```python
from build123d import *

# Parameters (mm, degrees)
F0_W      = 177.038
F0_H      = 34.544
F1_DEPTH  = 6.35
F2_R      = 6.35
F3_DEPTH  = 6.351
F4_DEPTH  = 25.4
F6_W      = 130.2497221681
F6_H      = 6.35
F6_W_2    = 46.7882778319
F7_DEPTH  = 7.874
F9_DEPTH  = 25.4
F11_DEPTH = 25.4


with BuildPart() as f1:
    # F0 (on Front) → F1 (new body)
    with BuildSketch(Plane.XZ):
        with Locations((88.519, 17.272)):
            Rectangle(F0_W, F0_H)
    extrude(amount=F1_DEPTH)

    # F2 (on face) → F3 (cut, through all)
    with BuildSketch(Plane.XZ.offset(6.35)):
        with Locations((28.448, 14.732)):
            Circle(F2_R)
    extrude(amount=-F3_DEPTH, mode=Mode.SUBTRACT)

    # F2 (on face) → F4 (cut)
    with BuildSketch(Plane.XZ.offset(6.35)):
        with Locations((28.448, 14.732)):
            Circle(F2_R)
        with Locations((76.2, 11.684)):
            Circle(F2_R)
        with Locations((136.144, 2.3622)):
            Circle(F2_R)
    extrude(amount=-F4_DEPTH, mode=Mode.SUBTRACT)

    # F6 (on face) → F7 (join)
    with BuildSketch(Plane(origin=(0, 0, 0), x_dir=(1, 0, 0), z_dir=(0, 0, -1))):
        with Locations((65.124861084, 3.175)):
            Rectangle(F6_W, F6_H)
        with Locations((153.643861084, 3.175)):
            Rectangle(F6_W_2, F6_H)
    extrude(amount=F7_DEPTH)

    # F8 (on face) → F9 (cut)
    with BuildSketch(Plane.XZ.offset(6.35)):
        with BuildLine():
            Line((142.0382778319, 0), (130.2497221681, 0))
            ThreePointArc((130.2497221681, 0), (136.144, -3.9878), (142.0382778319, 0))
        make_face()
    extrude(amount=-F9_DEPTH, mode=Mode.SUBTRACT)

    # F10 (on face) → F11 (cut)
    with BuildSketch(Plane.XZ.offset(6.35)):
        Polygon((167.894, 34.544), (9.144, 34.544), (9.144, 23.8669347018), (86.614, 23.8669347018), (86.614, 13.97), (167.894, 13.97), align=None)
        Polygon((61.8659904612, 4.6831931899), (0, 3.9632934857), (0, -7.874), (62.0121114495, -7.874), align=None)
    extrude(amount=-F11_DEPTH, mode=Mode.SUBTRACT)


solid = f1.part
```
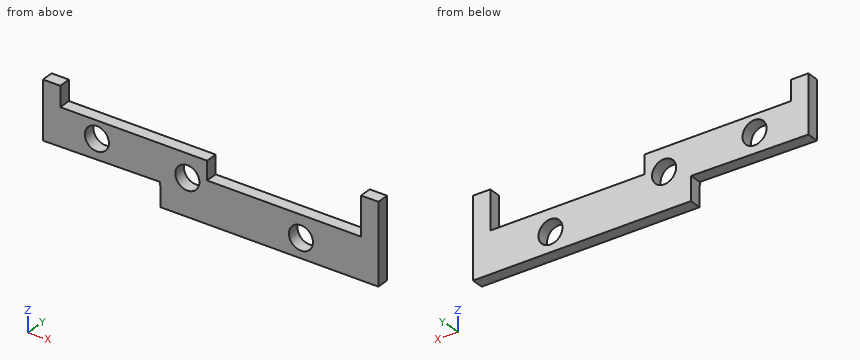
Geometry check sheet. Reference: the model listing, model coordinates, mm. Round coordinates to 2 decimals unless told otherwise and drop trailing zeros. Order: outer loops, then holes, each group sorted by start corner. A loop starts at its lowest first (then second) coordinate and runs counter-clockwise, first axis right, second up. Notation, with made-up numbers: (-14.75, -40) -> (0.25, -40) arc R24 cw to (0.25, -28) -> close; hole circle Ø7 at (42.25, 1.25). An arc over 180 degrees is marked (long way). Return JSON: item names as keys, results as strings. Group by question number.
Q1. Section check D-D, the plane x = 12.5. Record the boundary of the cut face in (y, z).
Q2. Section check C-C, the plane y = -3. Record the boundary of the cut face in (x, z).
Q3. Section check A-A, the plane z = 27.5. Record the boundary of the cut face in (x, y), plus the area to 3 significant figures.
Q4. Gauge pin test, flat ends, axial feed: pin 1 (3 mm diameter, centred on x = 81, y = -2, fed in from +Z); pin 2 (1.9 mm diameter, centred on x = 126, y = -4, fed in from +Z). Record the tip position at first contact, or that the pin passes through.
Q5. Material ranges on probe 1 along X at (y, z) = (-3.25, 27); probe 2 along X at (y, z) = (-3.5, 12); probe 3 along Z at (x, y) = (76.2, -2.25), recorded low to high. Write a range as from..to.
Q6. Section check B-B, the plane x = 76.2. Record the boundary of the cut face in (y, z).
Numbers:
{
 "1": {"outline": "(-6.35, 4.11) -> (0, 4.11) -> (0, 23.87) -> (-6.35, 23.87) -> close"},
 "2": {"outline": "(0, 3.96) -> (61.87, 4.68) -> (62.01, -7.87) -> (177.04, -7.87) -> (177.04, 34.54) -> (167.89, 34.54) -> (167.89, 13.97) -> (86.61, 13.97) -> (86.61, 23.87) -> (9.14, 23.87) -> (9.14, 34.54) -> (0, 34.54) -> close; hole circle Ø12.7 at (28.45, 14.73); hole circle Ø12.7 at (76.2, 11.68); hole circle Ø12.7 at (136.14, 2.36)"},
 "3": {"outline": "(0, -6.35) -> (9.14, -6.35) -> (9.14, 0) -> (0, 0) -> close; (167.89, -6.35) -> (177.04, -6.35) -> (177.04, 0) -> (167.89, 0) -> close", "area": "116 mm^2"},
 "4": {"pin 1": "z = 23.87", "pin 2": "z = 13.97"},
 "5": {"probe 1": "0..9.14, 167.89..177.04", "probe 2": "0..22.72, 34.18..69.86, 82.54..177.04", "probe 3": "-7.87..5.33, 18.03..23.87"},
 "6": {"outline": "(-6.35, -7.87) -> (0, -7.87) -> (0, 5.33) -> (-6.35, 5.33) -> close; (-6.35, 18.03) -> (0, 18.03) -> (0, 23.87) -> (-6.35, 23.87) -> close"}
}
